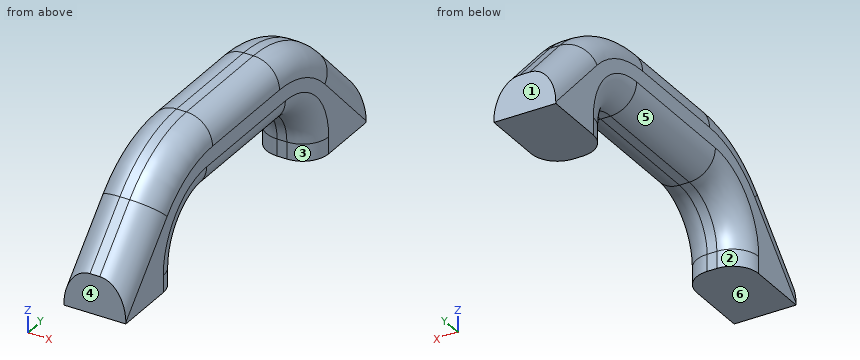
from build123d import *

# Parameters (mm, degrees)
F1_DEPTH      = 15.08125
F1_DEPTH_BACK = 15.08125
F2_R          = 63.5
F3_R          = 22.225
F4_R          = 12.7


with BuildPart() as f1:
    # F0 (on Right) → F1 (new body, two sides)
    with BuildSketch(Plane.YZ) as f1_sk:
        Polygon((0, 19.05), (0, 0), (42.8625, 0), (42.8625, 30.48), (96.8375, 30.48), (150.7998, 30.48), (150.7998, 0), (193.675, 0), (193.675, 19.05), (150.7998, 63.5), (42.8625, 63.5), align=None)
    extrude(amount=F1_DEPTH)
    extrude(f1_sk.sketch, amount=-F1_DEPTH_BACK)

    # F2
    f2_edges = [f1.edges().sort_by_distance(p)[0] for p in [
        (0, 42.8625, 63.5),
        (0, 150.7998, 63.5),
    ]]
    fillet(f2_edges, radius=F2_R)

    # F3
    f3_edges = [f1.edges().sort_by_distance(p)[0] for p in [
        (0, 42.8625, 30.48),
        (0, 150.7998, 30.48),
    ]]
    fillet(f3_edges, radius=F3_R)

    # F4
    f4_edges = [f1.edges().sort_by_distance(p)[0] for p in [
        (15.08125, 96.83115, 30.48),
        (-15.08125, 96.83115, 30.48),
        (-15.08125, 96.833924, 63.5),
        (15.08125, 96.833924, 63.5),
    ]]
    fillet(f4_edges, radius=F4_R)


solid = f1.part
Read the model definition and answer for the solid it produces. Units are mm, in the model's axes. Face numbers are marked on the shaded views. A direction names the side the tool comes from. Coordinates: 2 decimals unless noted, no trailing zeros. Order: outer loops, then holes, each group sorted by start corner. A loop starts at its lowest first (then second) coordinate and runs counter-clockwise, first axis right, second up. Notation, with made-up numbers: (10.25, -23) - (26.25, -23) arc R29 ccw to (26.25, -3) - close; hole circle Ø11 at (-11.5, 13.25). An arc over 180 degrees is marked (long way). Use one line per item in the form item = value.
(1) Which of the six approach directions +Z, -Z, +X, -X, +Y, -Y give full straight-line access (tool end or side, diameter ignored) to the marked faces 1, 2 and 3?
Computed values:
face_1 = +Z, -Z, +X, -X, +Y
face_2 = -Z, -X
face_3 = -Z, +X
(2) Straight lines are drawn through the part: L1, parallel to Z at x = 2.5, y = 94.5; L2, parallel to Y at x = -2.5, z = 14 (3 decimals); L3, parallel to X at y = 82.5, z = 60. For each, find the intervals that lie inside material, in ascending order.
Computed values:
L1 = 30.48 to 63.5
L2 = 0 to 43.617, 150.045 to 193.675
L3 = -11.14 to 11.14
(3) Section B-B, the plane x = 13 is taken. Give the vertices of the cut face in (y, z) (1 decimal), then the cut area to 3 significant figures.
Computed values:
outline = (0, 0) - (37.1, 0) - (37.1, 8.3) arc R28 cw to (65.1, 36.2) - (128.6, 36.2) arc R28 cw to (156.5, 8.3) - (156.5, 0) - (193.7, 0) - (193.7, 10.8) - (165.4, 40.1) arc R57.8 ccw to (123.8, 57.8) - (69.8, 57.8) arc R57.8 ccw to (28.3, 40.1) - (0, 10.8) - close
area = 4,920 mm²
(4) Given pin 1 Ø8 at (x, z) = (11, 28.5) entering from +Y; pin 2 Ø5 at (x, y) = (-1, 89) entering from -Z; pin 3 Ø5 at (x, z) = (-0.5, 3.5) entering from -Y; pin 4 Ø2 at (y, z) = (35, 49.5) entering from -X, each flat-ended and moving along its own axis, determine where each tip first touches the part or whether it passes through.
Computed values:
pin_1 = 185.39
pin_2 = 30.48
pin_3 = 0
pin_4 = -11.6
(5) For a pull along Y with two mould halves and no side action, classify the marked faces 4, 5 and 6 as pulls with the +Y half, pulls with the -Y half, needs draft (parallel to the pull), parting line crosses it, or undercut.
Computed values:
face_4 = pulls with the -Y half
face_5 = undercut
face_6 = needs draft
